```python
from build123d import *

# Parameters (mm, degrees)
EXTRU_MINCE1_DEPTH = 10
BOSS_EXTRU_1_DEPTH = 1


with BuildPart() as part:
    # Esquisse1 → Extru.-Mince1 (new body)
    with BuildSketch(Plane(origin=(0, 0, 0), x_dir=(1, 0, 0), z_dir=(0, 1, 0))):
        Polygon((225.762963936, -90.882191775), (27.185876504, -19.369864417), (27.185876504, 19.364097393), (225.762963936, 92.035383262), align=None)
        Polygon((224.262963936, -88.747703615), (28.685876504, -18.315747537), (28.685876504, 18.315747537), (224.262963936, 89.889153179), align=None, mode=Mode.SUBTRACT)
    extrude(amount=EXTRU_MINCE1_DEPTH)

    # Esquisse2 → Boss.-Extru.1 (add)
    with BuildSketch(Plane(origin=(0, 10, 0), x_dir=(1, 0, 0), z_dir=(0, 1, 0))):
        Polygon((225.762963936, -90.882191775), (225.762963936, 92.035383262), (27.185876504, 19.364097393), (27.185876504, -19.369864417), align=None)
    extrude(amount=BOSS_EXTRU_1_DEPTH)


solid = part.part
```
Source: CAD feature listing. Evaluate the final solid. Frame: model axes, mm. A direction names the side the tool comes from. Coordinates: 2 decimals unless noted, no trailing zeros. Loops run counter-clockwise (first coordinate to the right, second up) from the corner with the lowest first, then second, coordinate; pieces in that order, holes last. Notation, with made-up numbers: M 10.5,-3 L 46.5,-3 A25 ccw 46.5,34 Z; hole C -31,21.5 d4. An arc over 180 degrees is marked long. Use a Markdown table: item, result. Add a question column.
Q1. Section query A-A, the plane y = 4.5. Return loops of the section in (x, z).
Q2. Section query C-C, the plane x = 77.5. Return loops of the section in (y, z).
Q3. First-contact query: pin 1 (1.5 mm diameter, centred on x = 149, z = 25, fed in from -Y); pin 2 (4 mm diameter, centred on x = 112, y = 8, fed in from +Z). Flat tips, straight axial feed; report the tip coordinate or a pass-through.
Q4. Material intervals for L1, parallel to X at y = 2.5, z = -13; L2, parallel to Y at x = 120.5, z = 4; L3, parallel to Z at x = 211, y = 3, sorted ascending.
Q5. Draft query along X for faces 3 (the flat face through (147, 10, -2)), 4 (the flat face through (105, 0, 46)), 5 (the flat face through (125.084, 5.423, 54.625)). Return one class per face: pulls with the +X half, pulls with the -X half, needs draft (parallel to the pull), parting line crosses it, or undercut.
Q6. Section query B-B, the plane z = -4.5. Return loops of the section in (x, y).
Q7. Access query for faces 1 (the flat face through (127.864, 5.423, -56.208)), 2 (the flat face through (224.263, 5, -2)). Directions: +Z, -Z, +X, -X, +Y, -Y. A direction counts if a zero-diameter tool reaches every point of the face in a straight line with its end or side. Return the directions, or none.
Result:
| question | item | result |
|---|---|---|
| 1 | outline | M 27.19,-19.36 L 225.76,-92.04 L 225.76,90.88 L 27.19,19.37 Z; hole M 28.69,-18.32 L 224.26,-89.89 L 224.26,88.75 L 28.69,18.32 Z |
| 2 | outline | M 0,-37.78 L 11,-37.78 L 11,37.49 L 0,37.49 L 0,35.89 L 10,35.89 L 10,-36.18 L 0,-36.18 Z |
| 3 | pin 1 | stops at y = 10 |
| 3 | pin 2 | stops at z = 50.63 |
| 4 | L1 | x = 27.19 to 28.69, 224.26 to 225.76 |
| 4 | L2 | y = 10 to 11 |
| 4 | L3 | z = -86.63 to -85.04, 83.97 to 85.57 |
| 5 | face 3 | undercut |
| 5 | face 4 | needs draft |
| 5 | face 5 | pulls with the -X half |
| 6 | outline | M 27.19,0 L 28.69,0 L 28.69,10 L 224.26,10 L 224.26,0 L 225.76,0 L 225.76,11 L 27.19,11 Z |
| 7 | face 1 | -Z, -X, +Y, -Y |
| 7 | face 2 | -Y |
